Here's how the part is built. I have some questions about the finished solid (model axes, mm). Face numbers are marked on the shaded views. A direction names the side the tool comes from. Coordinates: 2 decimals unless noted, no trailing zeros. Loops run counter-clockwise (first coordinate to the right, second up) from the corner with the lowest first, then second, coordinate; pieces in that order, holes last.
from build123d import *

# Parameters (mm, degrees)
F1_DEPTH  = 5
F2_R      = 7.5
F3_W      = 6
F3_H      = 4
F3_W_2    = 3.5
F3_H_2    = 7
F4_DEPTH  = 17
F4_FACE_W = 3.5
F4_FACE_H = 7
F5_DEPTH  = 4


with BuildPart() as f1:
    # F0 (on Top) → F1 (new body)
    with BuildSketch(Plane.XY):
        Polygon((-35.669873, -20.594011), (35.669873, -20.594011), (0, 41.188022), align=None)
    extrude(amount=F1_DEPTH)

    # F2
    f2_edges = [f1.edges().sort_by_distance(p)[0] for p in [
        (35.669873, -20.594011, 2.5),
        (0, 41.188022, 2.5),
        (-35.669873, -20.594011, 2.5),
    ]]
    fillet(f2_edges, radius=F2_R)

    # F3 (on face) → F4 (join)
    with BuildSketch(Plane.XY.offset(5)):
        with Locations((-11, -7.906166)):
            Rectangle(F3_W, F3_H)
        with Locations((11, -7.906166)):
            Rectangle(F3_W, F3_H)
        with Locations((0, 14.593834)):
            Rectangle(F3_W_2, F3_H_2)
    extrude(amount=F4_DEPTH)

    # F4_face (on face) → F5 (join)
    with BuildSketch(Plane(origin=(0, 14.593834, 22), x_dir=(1, 0, 0), z_dir=(0, 0, 1))):
        Rectangle(F4_FACE_W, F4_FACE_H)
    extrude(amount=F5_DEPTH)


solid = f1.part
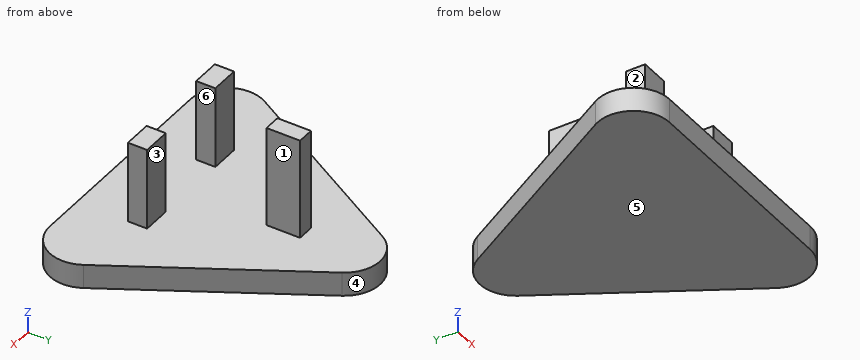
Q1. Will these pins go through, and if not, where does the flat tip stop? P1, Ø6, axis at x = 21.5, z = 10, coming from the -Y side; P2, Ø1.2, axis at y = -8.5, z = 16, coming from the -X side; P3, Ø1.5, axis at y = 17, z = 6, coming from the -X side; P4, Ø1, axis at x = -0.5, z = 14, coming from the +Y side.
Q2. Please list where these lines run through material, in increasing order: probe 1 along X at (y, z) = (-9, 21.75); probe 2 along Z at (x, y) = (-23, -15.5); probe 3 along Y at (x, z) = (12, 18.5).
Q3. Suppose I cut it at A-A on z = 20.25. Write out the boundary of the cut face in (x, y), and give its area (3 significant figures).
Q4. For the marked faces 1, 2 and 3, which set-ups out of +Z, -Z, +X, -X, +Y, -Y let a thin tool reach every point of the face, with its end or its side?
Q5. Suppose I cut it at C-C on x = 12. Write out the boundary of the cut face in (y, z).
Q6. Suppose I cut it at B-B on z = 2.5. Write out the boundary of the cut face in (x, y).
Q7. We'd pull the mould along X, two halves only. Please class the marked faces 4, 5 and 6: pulls with the +X half, pulls with the -X half, needs draft (parallel to the pull), parting line crosses it, or undercut.
Q8. Suppose I cut it at D-D on y = 13. Write out the boundary of the cut face in (x, z).
Check values:
1. P1: passes through
1. P2: stops at x = -14
1. P3: stops at x = -1.75
1. P4: stops at y = 18.09
2. probe 1: x = -14 to -8, 8 to 14
2. probe 2: z = 0 to 5
2. probe 3: y = -9.91 to -5.91
3. outline: (-14, -9.91) - (-8, -9.91) - (-8, -5.91) - (-14, -5.91) - close; (-1.75, 11.09) - (1.75, 11.09) - (1.75, 18.09) - (-1.75, 18.09) - close; (8, -9.91) - (14, -9.91) - (14, -5.91) - (8, -5.91) - close
3. area: 72.5 mm2
4. face 1: +Z, +X, +Y, -Y
4. face 2: +Z, -X, +Y, -Y
4. face 3: +Z, +X, -X, +Y
5. outline: (-20.59, 0) - (20.4, 0) - (20.4, 5) - (-5.91, 5) - (-5.91, 22) - (-9.91, 22) - (-9.91, 5) - (-20.59, 5) - close
6. outline: (-29.17, -9.34) arc R7.5 ccw to (-22.68, -20.59) - (22.68, -20.59) arc R7.5 ccw to (29.17, -9.34) - (6.5, 29.94) arc R7.5 ccw to (-6.5, 29.94) - close
7. face 4: parting line crosses it
7. face 5: needs draft
7. face 6: undercut
8. outline: (-16.27, 0) - (16.27, 0) - (16.27, 5) - (1.75, 5) - (1.75, 26) - (-1.75, 26) - (-1.75, 5) - (-16.27, 5) - close
